Verification items for this drawing (mm, ordinates from the low corner). Round coordinates to 2 decimals unless told otherwise and drop trailing zeros. Order: outer loops, then holes, each group sorted by start corner. A loop starts at its lowest first (then second) coordinate and runs counter-clockwise, first axis right, second up.
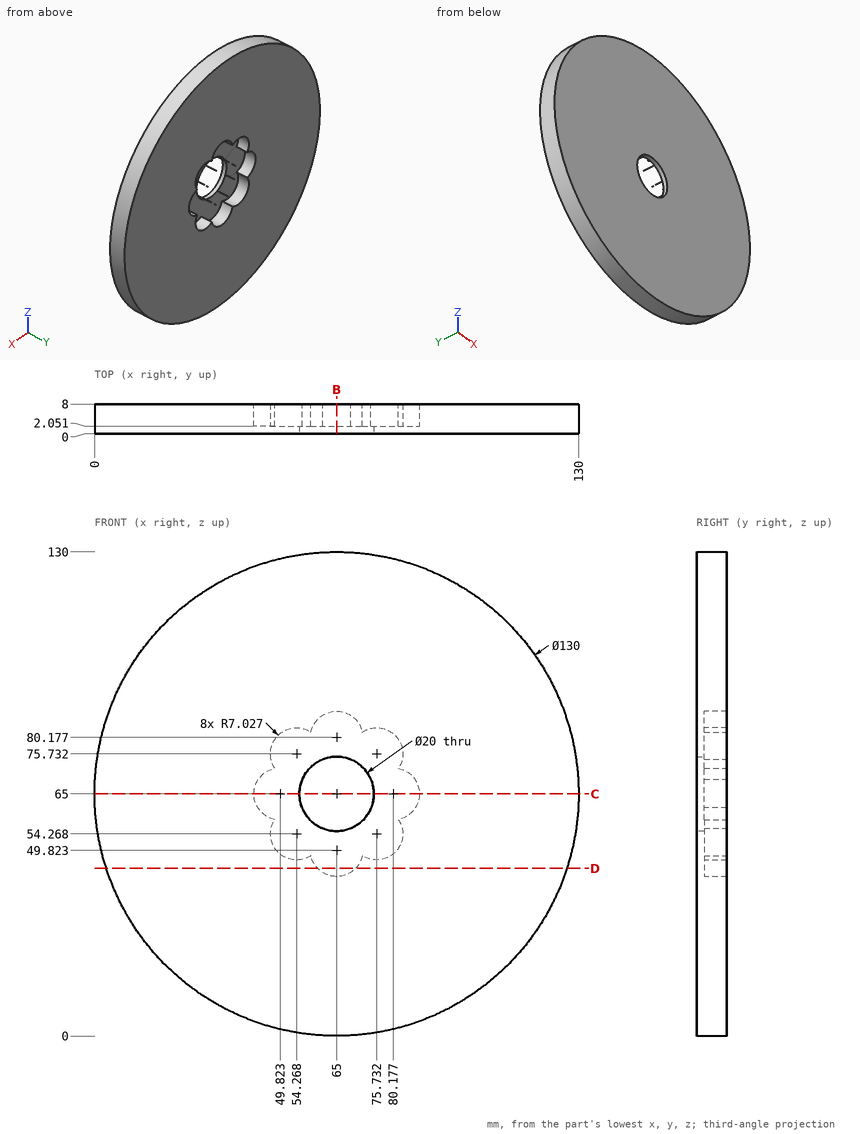
Item 1: Scan lines: line 1 along Z through (x, y) = (83, 6.75) (1 decimal); line 2 along X through (y, z) = (5.75, 76.5) (1 decimal); line 3 along X through (y, z) = (4, 78.5). Record each from-to range of solid material in increasing order.
Answer:
line 1: z = 2.5 to 58.6, 71.4 to 127.5
line 2: x = 1 to 47.3, 82.7 to 129
line 3: x = 1.42 to 47.81, 82.19 to 128.58
Item 2: Sectioned sample at B-B (x = 65). Record the cut outline in (y, z).
Answer:
outline: (0, 0) - (8, 0) - (8, 42.8) - (2.05, 42.8) - (2.05, 55) - (0, 55) - close; (0, 75) - (2.05, 75) - (2.05, 87.2) - (8, 87.2) - (8, 130) - (0, 130) - close
Item 3: Sectioned sample at C-C (z = 65). Record the cut outline in (x, y).
Answer:
outline: (0, 0) - (55, 0) - (55, 2.05) - (42.8, 2.05) - (42.8, 8) - (0, 8) - close; (75, 0) - (130, 0) - (130, 8) - (87.2, 8) - (87.2, 2.05) - (75, 2.05) - close
Item 4: Go/stop test with flat-tipped pins: P1, Ø4, axis at x = 27, y = 3, coming from the -Z side; P2, Ø4, axis at y = 6, z = 48.5, coming from the -X side; P3, Ø3, axis at x = 58.5, y = 4, coming from the -Z side; P4, Ø18, axis at x = 65, z = 65, coming from the -Y side. Record where each tip stops, or that it passes through.
Answer:
P1: stops at z = 10.88
P2: stops at x = 1.64
P3: stops at z = 0.19
P4: passes through
Item 5: Sectioned sample at D-D (z = 45). Record the cut outline in (x, y).
Answer:
outline: (3.15, 0) - (126.85, 0) - (126.85, 8) - (70.11, 8) - (70.11, 2.05) - (59.89, 2.05) - (59.89, 8) - (3.15, 8) - close
